```python
from build123d import *

# Parameters (mm, degrees)
BOSS_EXTRUDE1_DEPTH = 19
BOSS_EXTRUDE2_DEPTH = 9
FILLET5_R           = 3
CUT_EXTRUDE2_REACH  = 83.322
FILLET6_R           = 3


with BuildPart() as part:
    # Sketch1 → Boss-Extrude1 (new, symmetric)
    with BuildSketch(Plane.XY):
        with BuildLine():
            ThreePointArc((27, 0), (0, -27), (-27, 0))
            Line((-27, 0), (-36, 0))
            ThreePointArc((-36, 0), (0, -36), (36, 0))
            Line((36, 0), (27, 0))
        make_face()
    extrude(amount=BOSS_EXTRUDE1_DEPTH, both=True)

    # Sketch1<3> → Boss-Extrude2 (add, symmetric)
    with BuildSketch(Plane.XY):
        Polygon((-51.5, 0), (-39, 0), (-39, -50), (-51.5, -40), align=None)
        Polygon((39, -50), (51.5, -40), (51.5, 0), (39, 0), align=None)
        with BuildLine():
            ThreePointArc((36, 0), (0, -36), (-36, 0))
            Line((-36, 0), (-39, 0))
            Line((-39, 0), (-39, -50))
            Line((-39, -50), (-26.5, -60))
            Line((-26.5, -60), (26.5, -60))
            Line((26.5, -60), (39, -50))
            Line((39, -50), (39, 0))
            Line((39, 0), (36, 0))
        make_face()
    extrude(amount=BOSS_EXTRUDE2_DEPTH, both=True)

    # Fillet5
    fillet5_edges = [part.edges().sort_by_distance(p)[0] for p in [
        (0, -36, -9),
        (0, -36, 9),
    ]]
    fillet(fillet5_edges, radius=FILLET5_R)

    # Sketch2 → Cut-Extrude2 (cut, up to next)
    with BuildSketch(Plane(origin=(0, 0, 0), x_dir=(1, 0, 0), z_dir=(0, 1, 0)), mode=Mode.PRIVATE) as cut_extrude2_sk1:
        with BuildLine():
            Line((-39, 4.387482194), (-39, 9))
            Line((-39, 9), (-51.5, 9))
            Line((-51.5, 9), (-51.5, -9))
            Line((-51.5, -9), (-39, -9))
            Line((-39, -9), (-39, -4.387482194))
            ThreePointArc((-39, -4.387482194), (-42.5, 0), (-39, 4.387482194))
        make_face()
    cut_extrude2_tool1 = extrude(cut_extrude2_sk1.sketch, amount=-CUT_EXTRUDE2_REACH, mode=Mode.PRIVATE) & part.part
    # Sketch2 → Cut-Extrude2 (cut, up to next)
    with BuildSketch(Plane(origin=(0, 0, 0), x_dir=(1, 0, 0), z_dir=(0, 1, 0)), mode=Mode.PRIVATE) as cut_extrude2_sk2:
        with BuildLine():
            Line((51.5, 9), (39, 9))
            Line((39, 9), (39, 4.387482194))
            ThreePointArc((39, 4.387482194), (42.5, 0), (39, -4.387482194))
            Line((39, -4.387482194), (39, -9))
            Line((39, -9), (51.5, -9))
            Line((51.5, -9), (51.5, 9))
        make_face()
    cut_extrude2_tool2 = extrude(cut_extrude2_sk2.sketch, amount=-CUT_EXTRUDE2_REACH, mode=Mode.PRIVATE) & part.part
    # Sketch2 → Cut-Extrude2 (cut, up to next)
    with BuildSketch(Plane(origin=(0, 0, 0), x_dir=(1, 0, 0), z_dir=(0, 1, 0)), mode=Mode.PRIVATE) as cut_extrude2_sk3:
        with BuildLine():
            ThreePointArc((40.25, 0), (39.912132318, 1.185854123), (39, 2.015564437))
            Line((39, 2.015564437), (39, -2.015564437))
            ThreePointArc((39, -2.015564437), (39.912132318, -1.185854123), (40.25, 0))
        make_face()
    cut_extrude2_tool3 = extrude(cut_extrude2_sk3.sketch, amount=-CUT_EXTRUDE2_REACH, mode=Mode.PRIVATE) & part.part
    # Sketch2 → Cut-Extrude2 (cut, up to next)
    with BuildSketch(Plane(origin=(0, 0, 0), x_dir=(1, 0, 0), z_dir=(0, 1, 0)), mode=Mode.PRIVATE) as cut_extrude2_sk4:
        with BuildLine():
            Line((39, -2.015564437), (39, 2.015564437))
            ThreePointArc((39, 2.015564437), (35.75, 0), (39, -2.015564437))
        make_face()
    cut_extrude2_tool4 = extrude(cut_extrude2_sk4.sketch, amount=-CUT_EXTRUDE2_REACH, mode=Mode.PRIVATE) & part.part
    # Sketch2 → Cut-Extrude2 (cut, up to next)
    with BuildSketch(Plane(origin=(0, 0, 0), x_dir=(1, 0, 0), z_dir=(0, 1, 0)), mode=Mode.PRIVATE) as cut_extrude2_sk5:
        with BuildLine():
            ThreePointArc((-35.75, 0), (-36.814145877, 1.912132318), (-39, 2.015564437))
            Line((-39, 2.015564437), (-39, -2.015564437))
            ThreePointArc((-39, -2.015564437), (-36.814145877, -1.912132318), (-35.75, 0))
        make_face()
    cut_extrude2_tool5 = extrude(cut_extrude2_sk5.sketch, amount=-CUT_EXTRUDE2_REACH, mode=Mode.PRIVATE) & part.part
    # Sketch2 → Cut-Extrude2 (cut, up to next)
    with BuildSketch(Plane(origin=(0, 0, 0), x_dir=(1, 0, 0), z_dir=(0, 1, 0)), mode=Mode.PRIVATE) as cut_extrude2_sk6:
        with BuildLine():
            Line((-39, -2.015564437), (-39, 2.015564437))
            ThreePointArc((-39, 2.015564437), (-40.25, 0), (-39, -2.015564437))
        make_face()
    cut_extrude2_tool6 = extrude(cut_extrude2_sk6.sketch, amount=-CUT_EXTRUDE2_REACH, mode=Mode.PRIVATE) & part.part
    # Sketch2 → Cut-Extrude2 (cut, up to next)
    with BuildSketch(Plane(origin=(0, 0, 0), x_dir=(1, 0, 0), z_dir=(0, 1, 0)), mode=Mode.PRIVATE) as cut_extrude2_sk7:
        with BuildLine():
            ThreePointArc((-35.75, 0), (-36.814145877, 1.912132318), (-39, 2.015564437))
            Line((-39, 2.015564437), (-39, -2.015564437))
            ThreePointArc((-39, -2.015564437), (-36.814145877, -1.912132318), (-35.75, 0))
        make_face()
    cut_extrude2_tool7 = extrude(cut_extrude2_sk7.sketch, amount=-CUT_EXTRUDE2_REACH, mode=Mode.PRIVATE) & part.part
    # Sketch2 → Cut-Extrude2 (cut, up to next)
    with BuildSketch(Plane(origin=(0, 0, 0), x_dir=(1, 0, 0), z_dir=(0, 1, 0)), mode=Mode.PRIVATE) as cut_extrude2_sk8:
        with BuildLine():
            Line((-39, -2.015564437), (-39, 2.015564437))
            ThreePointArc((-39, 2.015564437), (-40.25, 0), (-39, -2.015564437))
        make_face()
    cut_extrude2_tool8 = extrude(cut_extrude2_sk8.sketch, amount=-CUT_EXTRUDE2_REACH, mode=Mode.PRIVATE) & part.part
    # Sketch2 → Cut-Extrude2 (cut, up to next)
    with BuildSketch(Plane(origin=(0, 0, 0), x_dir=(1, 0, 0), z_dir=(0, 1, 0)), mode=Mode.PRIVATE) as cut_extrude2_sk9:
        with BuildLine():
            ThreePointArc((40.25, 0), (39.912132318, 1.185854123), (39, 2.015564437))
            Line((39, 2.015564437), (39, -2.015564437))
            ThreePointArc((39, -2.015564437), (39.912132318, -1.185854123), (40.25, 0))
        make_face()
    cut_extrude2_tool9 = extrude(cut_extrude2_sk9.sketch, amount=-CUT_EXTRUDE2_REACH, mode=Mode.PRIVATE) & part.part
    # Sketch2 → Cut-Extrude2 (cut, up to next)
    with BuildSketch(Plane(origin=(0, 0, 0), x_dir=(1, 0, 0), z_dir=(0, 1, 0)), mode=Mode.PRIVATE) as cut_extrude2_sk10:
        with BuildLine():
            Line((39, -2.015564437), (39, 2.015564437))
            ThreePointArc((39, 2.015564437), (35.75, 0), (39, -2.015564437))
        make_face()
    cut_extrude2_tool10 = extrude(cut_extrude2_sk10.sketch, amount=-CUT_EXTRUDE2_REACH, mode=Mode.PRIVATE) & part.part
    add(cut_extrude2_tool1.solids().sort_by_distance((-45.792249, 0, 0))[0], mode=Mode.SUBTRACT)
    add(cut_extrude2_tool2.solids().sort_by_distance((45.792249, 0, 0))[0], mode=Mode.SUBTRACT)
    add(cut_extrude2_tool3.solids().sort_by_distance((39.51422, 0, 0))[0], mode=Mode.SUBTRACT)
    add(cut_extrude2_tool4.solids().sort_by_distance((37.556167, 0, 0))[0], mode=Mode.SUBTRACT)
    add(cut_extrude2_tool5.solids().sort_by_distance((-37.556167, 0, 0))[0], mode=Mode.SUBTRACT)
    add(cut_extrude2_tool6.solids().sort_by_distance((-39.51422, 0, 0))[0], mode=Mode.SUBTRACT)
    add(cut_extrude2_tool7.solids().sort_by_distance((-37.556167, 0, 0))[0], mode=Mode.SUBTRACT)
    add(cut_extrude2_tool8.solids().sort_by_distance((-39.51422, 0, 0))[0], mode=Mode.SUBTRACT)
    add(cut_extrude2_tool9.solids().sort_by_distance((39.51422, 0, 0))[0], mode=Mode.SUBTRACT)
    add(cut_extrude2_tool10.solids().sort_by_distance((37.556167, 0, 0))[0], mode=Mode.SUBTRACT)

    # Fillet6
    fillet6_edges = [part.edges().sort_by_distance(p)[0] for p in [
        (-39, -25, 4.387482194),
        (-39, -25, -4.387482194),
        (39, -25, -4.387482194),
        (39, -25, 4.387482194),
    ]]
    fillet(fillet6_edges, radius=FILLET6_R)


solid = part.part
```
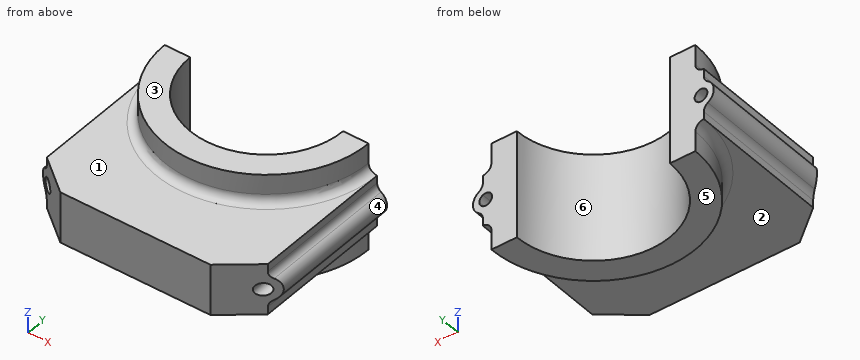
Source: CAD feature listing. Evaluate the final solid. Frame: model axes, mm. Face numbers are marked on the shaded views. A direction names the side the tool comes from. Coordinates: 2 decimals unless noted, no trailing zeros. Loops run counter-clockwise (first coordinate to the right, second up) from the corner with the lowest first, then second, coordinate; pieces in that order, holes last. Notation, with made-up numbers: M 43.25,28.5 L 71.25,28.5 A24 cw 71.25,45.5 Z; hole C 63.5,52 d6. An arc over 180 degrees is marked long. Put each result on its own line as item: value. Start each with the question number.
1) Pull-direction query (X, two-part tool) for the marked faces 4, 5 and 6; classes: pulls with the +X half, pulls with the -X half, needs draft (parallel to the pull), parting line crosses it, or undercut.
2) Cut plane C-C on x = 0. Return the cut outline in (y, z), then the cut area to 3 significant figures.
3) Contact query for flat-ended pins moving along their axis: pin 1 Ø0.8 at (y, z) = (-23, 8) entering from +X; pin 2 Ø12 at (x, y) = (-26.5, -44) entering from -Z; pin 3 Ø2 at (y, z) = (-15.5, -7) entering from -X. Output: stop coordinate, or through.
4) Cut plane B-B on y = -13. Give the number of separate pieces and of enclosed holes in the cut face, then the cut area to 3 significant figures.
5) Ray query, L1, parallel to Z at x = 38, y = -31; L2, parallel to X at y = -47, z = -1.5; L3, parallel to Z at x = 27, y = -35.5. Return the intervals inside material, ascending. Write a range as from..to.
6) Cut plane A-A on z = 7.5. Return the cut outline in (x, y), then the cut area to 3 significant figures.
7) Reachability of the marked faces 1, 2 and 3 from +Z, -Z, +X, -X, +Y, -Y: full face, straight path, thin tool, end or side. Return the list, or none.
The answers:
1. face 4: pulls with the +X half
1. face 5: needs draft
1. face 6: undercut
2. outline: M -60,-9 L -39,-9 A3 cw -36,-12 L -36,-19 L -27,-19 L -27,19 L -36,19 L -36,12 A3 cw -39,9 L -60,9 Z
2. area: 778 mm²
3. pin 1: stops at x = 39
3. pin 2: stops at z = -9
3. pin 3: stops at x = -39.02
4. separate pieces: 2
4. enclosed holes: 2
4. area: 973 mm²
5. L1: z = -9..-2.25, 2.25..9
5. L2: x = -42.24..-39.68, -36.32..36.32, 39.68..42.24
5. L3: z = -9..9
6. outline: M -39,-50 L -26.5,-60 L 26.5,-60 L 39,-50 L 39,0 L 27,0 A27 cw -27,0 L -39,0 Z
6. area: 3,410 mm²
7. face 1: +Z, -Y
7. face 2: -Z, -Y
7. face 3: +Z, +X, -X, +Y, -Y
